Part model, mm, in its own coordinate system. Coordinates: 2 decimals unless noted, no trailing zeros. Order: outer loops, then holes, each group sorted by start corner. A loop starts at its lowest first (then second) coordinate and runs counter-clockwise, first axis right, second up.
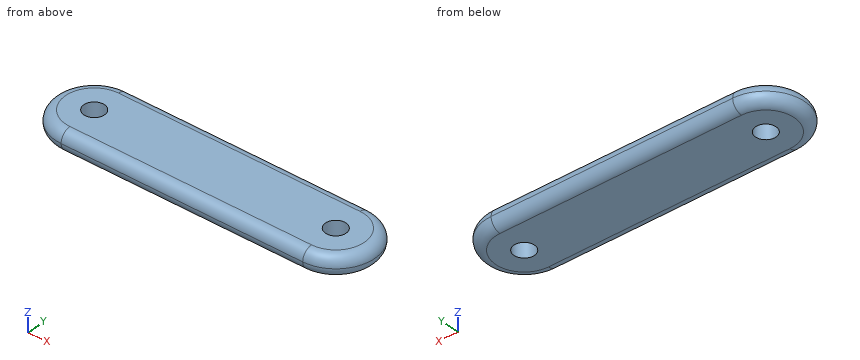
```python
from build123d import *

# Parameters (mm, degrees)
BOSS_EXTRUDE1_DEPTH         = 6.35
F_1_4_0_25_DIAMETER_HOLE1_D = 6.35
FILLET1_R                   = 3.175


with BuildPart() as part:
    # Sketch1 → Boss-Extrude1 (new body)
    with BuildSketch(Plane.XY):
        with BuildLine():
            Line((-37.000000041, 11.999999876), (37.000000041, 11.999999876))
            ThreePointArc((37.000000041, 11.999999876), (48.999999917, 0), (37.000000041, -11.999999876))
            Line((37.000000041, -11.999999876), (-37.000000041, -11.999999876))
            ThreePointArc((-37.000000041, -11.999999876), (-48.999999917, 0), (-37.000000041, 11.999999876))
        make_face()
    extrude(amount=BOSS_EXTRUDE1_DEPTH)

    # 1/4 (0.25) Diameter Hole1 (through all)
    with Locations(Plane.XY.offset(6.35)):
        with Locations((-37.000000041, 0), (37.000000041, 0)):
            Hole(F_1_4_0_25_DIAMETER_HOLE1_D / 2)

    # Fillet1
    fillet1_edges = [part.edges().sort_by_distance(p)[0] for p in [
        (48.999999917, 0, 6.35),
        (0, 11.999999876, 6.35),
        (-48.999999917, 0, 6.35),
        (0, 11.999999876, 0),
        (0, -11.999999876, 0),
        (0, -11.999999876, 6.35),
    ]]
    fillet(fillet1_edges, radius=FILLET1_R - 0.0001)  # a hair under: the kernel refuses the full size


solid = part.part
```
(1) Drop flat-ended pins along their axis: pin 1 (1 mm diameter, centred on x = -25.5, z = 3.5, fed in from +Y); pin 2 (1.5 mm diameter, centred on x = 30.5, z = 1.5, fed in from +Y); pin 3 (1.5 mm diameter, centred on x = -25, z = 1, fed in from -Y). Give the stop position or say it passes through.
(2) Slice it at C-C, the plane z = 5.5. Give the cut face in (x, y) (3 decimals).
(3) Probe line 1 (X direction, y = 0.5, z = 0.75); line 2 (Y direction, x = -37, z = 4.5) (3 decimals); line 3 (Y direction, x = 27, z = 3.25). List the from-to ranges inside material, lowest first.
(4) Slice it at A-A, the plane y = 0. State how many separate pieces and enclosed holes the cut face has, then the cut area to 3 significant figures.
Here are the results:
1. pin 1: stops at y = 12
1. pin 2: stops at y = 11.86
1. pin 3: stops at y = -11.66
2. outline: (-37, -10.987) - (37, -10.987) arc R10.987 ccw to (37, 10.987) - (-37, 10.987) arc R10.987 ccw to start; hole circle Ø6.35 at (-37, 0); hole circle Ø6.35 at (37, 0)
3. line 1: x = -47.86 to -40.14, -33.86 to 33.86, 40.14 to 47.86
3. line 2: y = -11.71 to -3.175, 3.175 to 11.71
3. line 3: y = -12 to 12
4. separate pieces: 3
4. enclosed holes: 0
4. area: 533 mm2
